Geometry: final body of the model. Coordinates: model frame, mm. Coordinates: 2 decimals unless noted, no trailing zeros. Order: outer loops, then holes, each group sorted by start corner. A loop starts at its lowest first (then second) coordinate and runs counter-clockwise, first axis right, second up. Notation, with made-up numbers: M 75.25,15 L 101.25,15 A17 cw 101.25,42 Z; hole C -5,-23 d3. An arc over 180 degrees is marked long. Use CSV: the item, a comma, the result in double quotes. Start each with the question number.
Q1. Ray query, probe 1 along Y at (x, z) = (206.15, 2.45); probe 2 along Y at (x, z) = (147.5, 4.4); probe 3 along Y at (x, z) = (-3.5, 4.1). Return the intervals inside material, ascending.
Q2. First-contact query: P1, Ø5, axis at x = -153.5, y = -25.5, coming from the -Z side. Flat tip, straight axial feed; report the tip coordinate or a pass-through.
Q3. Section query B-B, the plane z = 3.3. State how many separate pieces and enclosed holes the cut face has, and give its area (3 significant figures).
Q4. Section query A-A, the plane x = 55. Output: boundary loops of the cut face in (y, z), and give its area (3 significant figures).
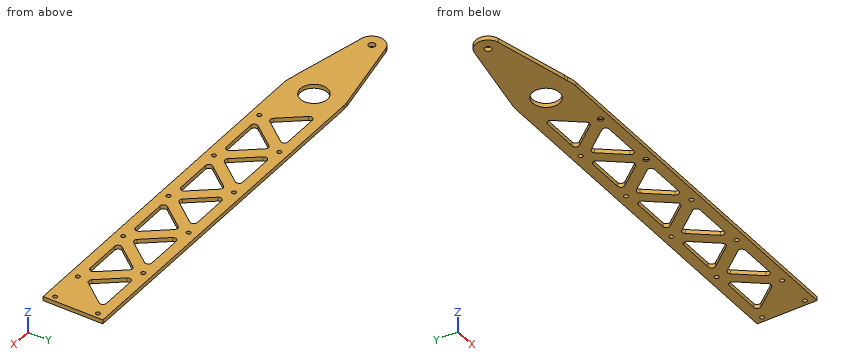
from build123d import *

# Parameters (mm, degrees)
SKETCH1_R                                       = 3.96875
SKETCH1_R_2                                     = 15.875
BOSS_EXTRUDE1_DEPTH                             = 4.7625
F_10_CLEARANCE_HOLE1_D                          = 4.9784
LPATTERN1_COUNT                                 = 4
LPATTERN1_PITCH                                 = 80
CUT_EXTRUDE1_DEPTH                              = 10
FILLET1_R                                       = 4
CUT_EXTRUDE2_DEPTH                              = 5.7625
FILLET2_R                                       = 4
LPATTERN2_COUNT                                 = 4
LPATTERN2_PITCH                                 = 80
FILLET1_OF_LPATTERN2_R                          = 4
LPATTERN3_COUNT                                 = 3
LPATTERN3_PITCH                                 = 80
FILLET2_OF_LPATTERN3_R                          = 4
LPATTERN4_COUNT                                 = 2
LPATTERN4_PITCH                                 = 80
FILLET2_OF_LPATTERN4_R                          = 4
LPATTERN5_COUNT                                 = 2
LPATTERN5_PITCH                                 = 80
FILLET1_OF_LPATTERN5_R                          = 4
F_10_CLEARANCE_HOLE2_D                          = 4.9784
F_10_CLEARANCE_HOLE2_DEPTH                      = 4.7625
CBORE_FOR_10_BUTTON_HEAD_CAP_SCREW1_D           = 4.9784
CBORE_FOR_10_BUTTON_HEAD_CAP_SCREW1_CBORE_D     = 6.35
CBORE_FOR_10_BUTTON_HEAD_CAP_SCREW1_CBORE_DEPTH = 1.5875


with BuildPart() as part:
    # Sketch1 → Boss-Extrude1 (new body)
    with BuildSketch(Plane.XY):
        with BuildLine():
            Line((212.5, 35), (-212.5, 35))
            ThreePointArc((-212.5, 35), (-215.694597401, 34.853902901), (-218.862525007, 34.416831283))
            Line((-218.862525007, 34.416831283), (-313.666145568, 16.890801601))
            ThreePointArc((-313.666145568, 16.890801601), (-325.748634462, 2.719438205), (-314.360273, -12.015530461))
            Line((-314.360273, -12.015530461), (-228.749110944, -32.134843328))
            Line((-228.749110944, -32.134843328), (-224.470705016, -32.889241728))
            ThreePointArc((-224.470705016, -32.889241728), (-218.577686218, -34.468271355), (-212.5, -35))
            Line((-212.5, -35), (212.5, -35))
            Line((212.5, -35), (212.5, 35))
        make_face()
        with Locations((-310.980775301, 2.364817767)):
            Circle(SKETCH1_R, mode=Mode.SUBTRACT)
        with Locations((-212.5, 0)):
            Circle(SKETCH1_R_2, mode=Mode.SUBTRACT)
    extrude(amount=BOSS_EXTRUDE1_DEPTH)

    # #10 Clearance Hole1 (through all)
    with Locations(Plane(origin=(0, 0, 0), x_dir=(-1, 0, 0), z_dir=(0, 0, -1))):
        with Locations((-126.15, 25), (-86.15, -25)):
            f_10_clearance_hole1 = Hole(F_10_CLEARANCE_HOLE1_D / 2)

    # LPattern1: #10 Clearance Hole1 ×4
    with Locations(*[(-i * LPATTERN1_PITCH, 0, 0) for i in range(1, LPATTERN1_COUNT)]):
        add(f_10_clearance_hole1, mode=Mode.SUBTRACT)

    # Sketch13 → Cut-Extrude1 (cut)
    with BuildSketch(Plane(origin=(0, 0, 0), x_dir=(-1, 0, 0), z_dir=(0, 0, -1))):
        Polygon((-56.301294523, 22.715958732), (-86.15, -14.594923114), (-115.998705477, 22.715958732), align=None)
    cut_extrude1 = extrude(amount=-CUT_EXTRUDE1_DEPTH, mode=Mode.SUBTRACT)

    # Fillet1
    fillet1_edges = [part.edges().sort_by_distance(p)[0] for p in [
        (56.301294523, 22.715958732, 2.38125),
        (86.15, -14.594923114, 2.38125),
        (115.998705477, 22.715958732, 2.38125),
    ]]
    fillet(fillet1_edges, radius=FILLET1_R)

    # Sketch14 → Cut-Extrude2 (cut, through all)
    with BuildSketch(Plane(origin=(0, 0, 0), x_dir=(-1, 0, 0), z_dir=(0, 0, -1))):
        Polygon((-46.15, 14.594923114), (-75.998705477, -22.715958732), (-16.301294523, -22.715958732), align=None)
    cut_extrude2 = extrude(amount=-CUT_EXTRUDE2_DEPTH, mode=Mode.SUBTRACT)

    # Fillet2
    fillet2_edges = [part.edges().sort_by_distance(p)[0] for p in [
        (46.15, 14.594923114, 2.38125),
        (16.301294523, -22.715958732, 2.38125),
        (75.998705477, -22.715958732, 2.38125),
    ]]
    fillet(fillet2_edges, radius=FILLET2_R)

    # LPattern2: Cut-Extrude1 ×4
    with Locations(*[(-i * LPATTERN2_PITCH, 0, 0) for i in range(1, LPATTERN2_COUNT)]):
        add(cut_extrude1, mode=Mode.SUBTRACT)

    # Fillet1 of LPattern2
    fillet1_of_lpattern2_edges = [part.edges().sort_by_distance(p)[0] for p in [
        (-23.698705477, 22.715958732, 2.38125),
        (6.15, -14.594923114, 2.38125),
        (35.998705477, 22.715958732, 2.38125),
        (-103.698705477, 22.715958732, 2.38125),
        (-73.85, -14.594923114, 2.38125),
        (-44.001294523, 22.715958732, 2.38125),
        (-183.698705477, 22.715958732, 2.38125),
        (-153.85, -14.594923114, 2.38125),
        (-124.001294523, 22.715958732, 2.38125),
    ]]
    fillet(fillet1_of_lpattern2_edges, radius=FILLET1_OF_LPATTERN2_R)

    # LPattern3: Cut-Extrude2 ×3
    with Locations(*[(-i * LPATTERN3_PITCH, 0, 0) for i in range(1, LPATTERN3_COUNT)]):
        add(cut_extrude2, mode=Mode.SUBTRACT)

    # Fillet2 of LPattern3
    fillet2_of_lpattern3_edges = [part.edges().sort_by_distance(p)[0] for p in [
        (-33.85, 14.594923114, 2.38125),
        (-63.698705477, -22.715958732, 2.38125),
        (-4.001294523, -22.715958732, 2.38125),
        (-113.85, 14.594923114, 2.38125),
        (-143.698705477, -22.715958732, 2.38125),
        (-84.001294523, -22.715958732, 2.38125),
    ]]
    fillet(fillet2_of_lpattern3_edges, radius=FILLET2_OF_LPATTERN3_R)

    # LPattern4: Cut-Extrude2 ×2
    with Locations(*[(i * LPATTERN4_PITCH, 0, 0) for i in range(1, LPATTERN4_COUNT)]):
        add(cut_extrude2, mode=Mode.SUBTRACT)

    # Fillet2 of LPattern4
    fillet2_of_lpattern4_edges = [part.edges().sort_by_distance(p)[0] for p in [
        (126.15, 14.594923114, 2.38125),
        (96.301294523, -22.715958732, 2.38125),
        (155.998705477, -22.715958732, 2.38125),
    ]]
    fillet(fillet2_of_lpattern4_edges, radius=FILLET2_OF_LPATTERN4_R)

    # LPattern5: Cut-Extrude1 ×2
    with Locations(*[(i * LPATTERN5_PITCH, 0, 0) for i in range(1, LPATTERN5_COUNT)]):
        add(cut_extrude1, mode=Mode.SUBTRACT)

    # Fillet1 of LPattern5
    fillet1_of_lpattern5_edges = [part.edges().sort_by_distance(p)[0] for p in [
        (136.301294523, 22.715958732, 2.38125),
        (166.15, -14.594923114, 2.38125),
        (195.998705477, 22.715958732, 2.38125),
    ]]
    fillet(fillet1_of_lpattern5_edges, radius=FILLET1_OF_LPATTERN5_R)

    # #10 Clearance Hole2
    with Locations(Plane.XY.offset(4.7625)):
        with Locations((206.15, 25), (206.15, -25), (166.15, -25)):
            Hole(F_10_CLEARANCE_HOLE2_D / 2, depth=F_10_CLEARANCE_HOLE2_DEPTH)

    # CBORE for #10 Button Head Cap Screw1 (through all)
    with Locations(Plane(origin=(0, 0, 0), x_dir=(-1, 0, 0), z_dir=(0, 0, -1))):
        with Locations((153.85, -25), (73.85, -25)):
            CounterBoreHole(CBORE_FOR_10_BUTTON_HEAD_CAP_SCREW1_D / 2, CBORE_FOR_10_BUTTON_HEAD_CAP_SCREW1_CBORE_D / 2, CBORE_FOR_10_BUTTON_HEAD_CAP_SCREW1_CBORE_DEPTH)


solid = part.part
Responses:
1,probe 1,"y = -35 to -27.49, -22.51 to 22.51, 27.49 to 35"
1,probe 2,"y = -35 to -22.72, -12.09 to 8.72, 22.72 to 35"
1,probe 3,"y = -35 to -2.53, 22.72 to 35"
2,P1,"stops at z = 1.59"
3,separate pieces,"1"
3,enclosed holes,"22"
3,area,"24,300 mm²"
4,outline,"M -35,0 L -22.72,0 L -22.72,4.76 L -35,4.76 Z; M 3.53,0 L 35,0 L 35,4.76 L 3.53,4.76 Z"
4,area,"208 mm²"
